from build123d import *

# Parameters (mm, degrees)
F0_R     = 1.65
F1_DEPTH = 1


with BuildPart() as f1:
    # F0 (on Top) → F1 (new body)
    with BuildSketch(Plane.XY):
        with BuildLine():
            Line((0, 74), (0, 0))
            Line((0, 0), (14, 0))
            ThreePointArc((14, 0), (15.414214, 0.585786), (16, 2))
            Line((16, 2), (16, 9.503425))
            ThreePointArc((16, 9.503425), (16.058935, 9.985367), (16.232268, 10.438906))
            Line((16.232268, 10.438906), (28.803195, 34.193557))
            ThreePointArc((28.803195, 34.193557), (29.5, 37), (28.803195, 39.806443))
            Line((28.803195, 39.806443), (16.232268, 63.561094))
            ThreePointArc((16.232268, 63.561094), (16.058935, 64.014633), (16, 64.496575))
            Line((16, 64.496575), (16, 72))
            ThreePointArc((16, 72), (15.414214, 73.414214), (14, 74))
            Line((14, 74), (0, 74))
        make_face()
        with Locations((23.5, 37)):
            Circle(F0_R, mode=Mode.SUBTRACT)
        with BuildLine():
            Line((-14, 0), (0, 0))
            Line((0, 0), (0, 74))
            Line((0, 74), (-14, 74))
            ThreePointArc((-14, 74), (-15.414214, 73.414214), (-16, 72))
            Line((-16, 72), (-16, 64.496575))
            ThreePointArc((-16, 64.496575), (-16.058935, 64.014633), (-16.232268, 63.561094))
            Line((-16.232268, 63.561094), (-28.803195, 39.806443))
            ThreePointArc((-28.803195, 39.806443), (-29.5, 37), (-28.803195, 34.193557))
            Line((-28.803195, 34.193557), (-16.232268, 10.438906))
            ThreePointArc((-16.232268, 10.438906), (-16.058935, 9.985367), (-16, 9.503425))
            Line((-16, 9.503425), (-16, 2))
            ThreePointArc((-16, 2), (-15.414214, 0.585786), (-14, 0))
        make_face()
        with Locations((-23.5, 37)):
            Circle(F0_R, mode=Mode.SUBTRACT)
    extrude(amount=F1_DEPTH)


solid = f1.part
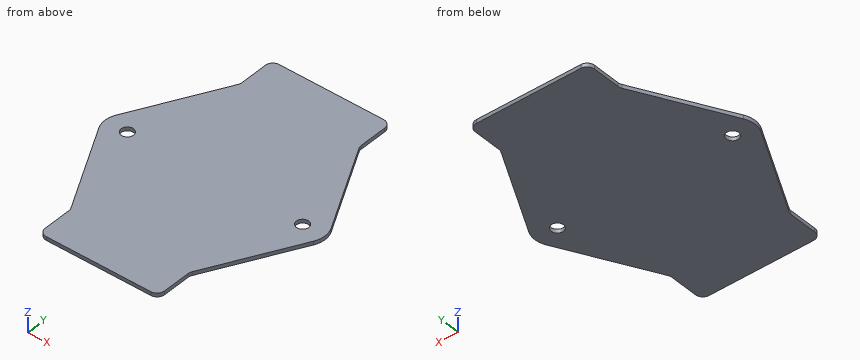
Design review of the part built by this model. Coordinates are the model's own, in mm. Round coordinates to 2 decimals unless told otherwise and drop trailing zeros. Loops run counter-clockwise (first coordinate to the right, second up) from the corner with the lowest first, then second, coordinate; pieces in that order, holes last. Notation, with made-up numbers: M -4,-17.5 L 27,-17.5 A27 cw 27,0.5 Z; hole C 23,61.5 d4. An arc over 180 degrees is marked long. Answer as a JSON object with one key per item and string values.
Item 1: We need section C-C on y = 6. Give the boundary of the cut face in (x, z).
Answer sheet:
{"outline": "M -16,0 L 16,0 L 16,1 L -16,1 Z"}
Item 2: We need section A-A on x = 23.5. Give the boundary of the cut face in (y, z).
Answer sheet:
{"outline": "M 24.17,0 L 35.35,0 L 35.35,1 L 24.17,1 Z; M 38.65,0 L 49.83,0 L 49.83,1 L 38.65,1 Z"}
Item 3: We need section D-D on x = -18. Give the boundary of the cut face in (y, z), and give its area (3 significant figures).
Answer sheet:
{"outline": "M 13.78,0 L 60.22,0 L 60.22,1 L 13.78,1 Z", "area": "46.4 mm^2"}
Item 4: We need section B-B on z = 0.45. Give the boundary of the cut face in (x, y), and give its area (3 significant figures).
Answer sheet:
{"outline": "M -28.8,34.19 L -16.23,10.44 A2 cw -16,9.5 L -16,2 A2 ccw -14,0 L 14,0 A2 ccw 16,2 L 16,9.5 A2 cw 16.23,10.44 L 28.8,34.19 A6 ccw 28.8,39.81 L 16.23,63.56 A2 cw 16,64.5 L 16,72 A2 ccw 14,74 L -14,74 A2 ccw -16,72 L -16,64.5 A2 cw -16.23,63.56 L -28.8,39.81 A6 ccw Z; hole C -23.5,37 d3.3; hole C 23.5,37 d3.3", "area": "3,120 mm^2"}
Item 5: Clearance check with flat-ended pins moving along their axes: P1, Ø4, axis at x = 23.5, y = 37, coming from the +Z side; P2, Ø0.5, axis at y = 69, z = 0.5, coming from the -X side. State where each tip first meets the part, or that it passes through.
Answer sheet:
{"P1": "stops at z = 1", "P2": "stops at x = -16"}
Item 6: Wall thickness on L1, parallel to X at y = 38.5, z = 0.45; L2, parallel to Y at x = -23.5, z = 0.8; L3, parallel to X at y = 6, z = 0.35: over which ranges is each line inside the solid? List them lowest first. Write a range as from..to.
Answer sheet:
{"L1": "x = -29.31..-24.19, -22.81..22.81, 24.19..29.31", "L2": "y = 24.17..35.35, 38.65..49.83", "L3": "x = -16..16"}
